Read the model definition and answer for the solid it produces. Units are mm, in the model's axes. A direction names the side the tool comes from. Round coordinates to 2 decimals unless told otherwise and drop trailing zeros. Loops run counter-clockwise (first coordinate to the right, second up) from the corner with the lowest first, then second, coordinate; pieces in that order, holes last. Notation, with made-up numbers: M -26,-27 L -5,-27 A27 ccw -5,7 Z; hole C -29.5,48.25 d2. An arc over 180 degrees is marked long. Answer as CSV lines item,"result".
```python
from build123d import *

# Parameters (mm, degrees)
BOSS_EXTRU_1_DEPTH      = 1
ESQUISSE2_W             = 4
ESQUISSE2_H             = 22.100446083
ENL_V_MAT_EXTRU_2_DEPTH = 0.5
ESQUISSE3_W             = 4
ESQUISSE3_H             = 22.262802535
BOSS_EXTRU_2_DEPTH      = 0.5
BOSS_EXTRU_2_DEPTH_BACK = 0.1


with BuildPart() as part:
    # Esquisse1 → Boss.-Extru.1 (new body)
    with BuildSketch(Plane.XY):
        Polygon((34.6, 20.706521175), (31.104320123, 20.706521175), (31.104320123, 23.497793163), (-33.095389285, 23.497793163), (-33.095389285, 8.252206837), (-34.510836618, 8.252206837), (-34.6, 8.252206837), (-34.6, -8.247793163), (-33.095389285, -8.247793163), (-33.095389285, -23.497793163), (31.104320123, -23.497793163), (31.104320123, -14.402052139), (34.6, -14.402052139), align=None)
    extrude(amount=BOSS_EXTRU_1_DEPTH)

    # Esquisse2 → Enlèv. mat.-Extru.2 (cut)
    with BuildSketch(Plane.XY.offset(1)):
        with Locations((32.6, -0.347632361)):
            Rectangle(ESQUISSE2_W, ESQUISSE2_H)
    extrude(amount=-ENL_V_MAT_EXTRU_2_DEPTH, mode=Mode.SUBTRACT)

    # Esquisse3 → Boss.-Extru.2 (add, two sides)
    with BuildSketch(Plane.XY.offset(1)) as boss_extru_2_sk:
        with Locations((32.6, -0.266454134)):
            Rectangle(ESQUISSE3_W, ESQUISSE3_H)
    extrude(amount=BOSS_EXTRU_2_DEPTH)
    extrude(boss_extru_2_sk.sketch, amount=-BOSS_EXTRU_2_DEPTH_BACK)


solid = part.part
```
1) Each of these flat-tipped pins is pushed along its axis until it touches: P1, Ø0.5, axis at x = 33, z = 0.5, coming from the +Y side; P2, Ø0.8, axis at y = 14, z = 0.5, coming from the -X side; P3, Ø8, axis at x = -4, y = 7.5, coming from the +Z side. Where does it stop, or does it pass through?
Evaluation:
P1,"stops at y = 20.71"
P2,"stops at x = -33.1"
P3,"stops at z = 1"
2) Determine the mould class of faces 1 (the flat face through (0, 0, 0)), 2 (the flat face through (33, 0, 0.9)), 3 (the flat face through (34.6, 2.9, 1.1)) for opening direction Z: released by +Z, released by -Z, zero draft, split by the parting line, or undercut.
Evaluation:
face 1,"released by -Z"
face 2,"undercut"
face 3,"zero draft"
3) A tool of negligible diameter and unlimited length cuts with its end or side. For faces 4 (the flat face through (33, 0, 0.5)), 5 (the flat face through (33, 0, 1.5)), from which of +Z, -Z, +X, -X, +Y, -Y can it reach the whole face along a straight path? Write none if from no direction.
Evaluation:
face 4,"+X"
face 5,"+Z, +X, -X, +Y, -Y"
4) Find section C-C, the plane x = 25.5. Give the vertices of the cut face in (y, z).
Evaluation:
outline,"M -23.5,0 L 23.5,0 L 23.5,1 L -23.5,1 Z"
5) Find section B-B, the plane z = 0.25. Give the vertices of the cut face in (x, y).
Evaluation:
outline,"M -34.6,-8.25 L -33.1,-8.25 L -33.1,-23.5 L 31.1,-23.5 L 31.1,-14.4 L 34.6,-14.4 L 34.6,20.71 L 31.1,20.71 L 31.1,23.5 L -33.1,23.5 L -33.1,8.25 L -34.6,8.25 Z"
6) Find section D-D, the plane y = 4. Give the vertices of the cut face in (x, z).
Evaluation:
outline,"M -34.6,0 L 34.6,0 L 34.6,0.5 L 30.6,0.5 L 30.6,0.9 L 34.6,0.9 L 34.6,1.5 L 30.6,1.5 L 30.6,1 L -34.6,1 Z"
7) Find section A-A, the plane y = 10. Give the vertices of the cut face in (x, z), then the cut area to 3 significant figures.
Evaluation:
outline,"M -33.1,0 L 34.6,0 L 34.6,0.5 L 30.6,0.5 L 30.6,0.9 L 34.6,0.9 L 34.6,1.5 L 30.6,1.5 L 30.6,1 L -33.1,1 Z"
area,"68.1 mm^2"
8) Straight lines are drawn through the part: line 1 (X direction, y = -14.5, z = 0.65); line 2 (Z direction, x = -18, y = -9); line 3 (X direction, y = 14.5, z = 0.1). For each, find the intervals that lie inside material, in ascending order.
Evaluation:
line 1,"x = -33.1 to 31.1"
line 2,"z = 0 to 1"
line 3,"x = -33.1 to 34.6"
